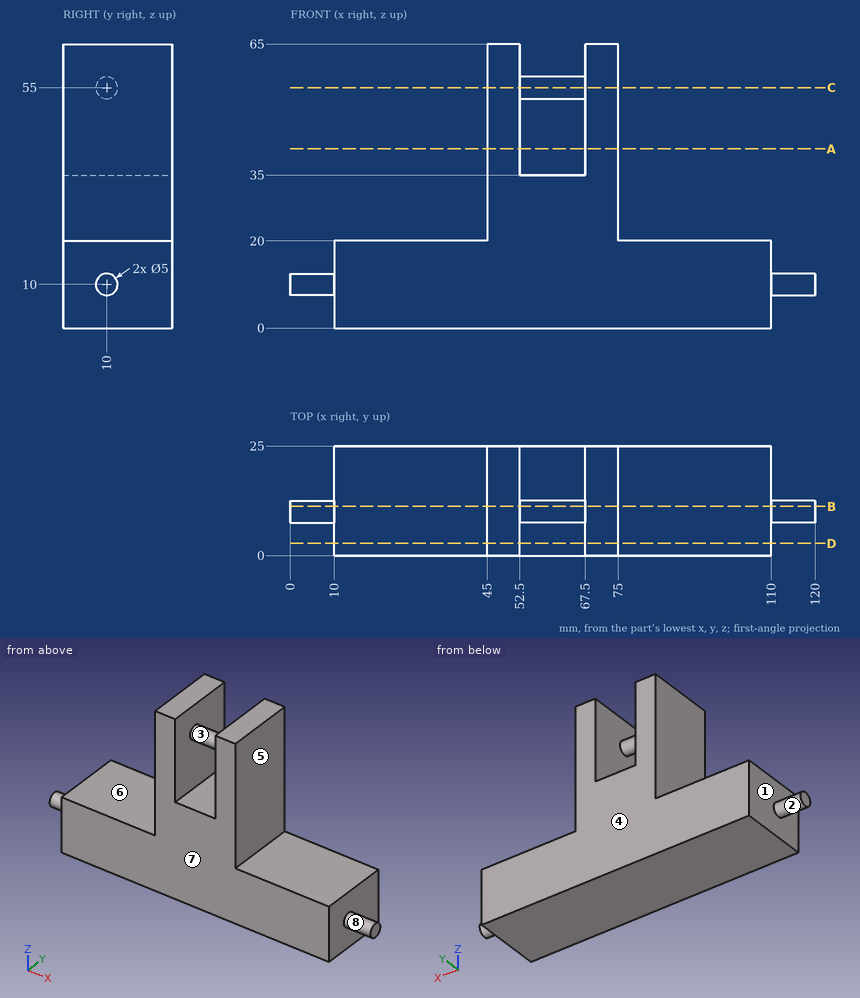
Answer from the drawing. Dimensions are ordinates in mm from the lowest x, y and z of the part. A direction names the side the tool comes from. Give positions to 0.01 mm unless a question says otherwise; leave off trailing zeros. Order: outer loops, then holes, each group sorted by start corner. A loop starts at its lowest first (then second) coordinate and runs counter-clockwise, first axis right, second up.
(1) Find section A-A (z = 41). Give the vertices of the cut face in (x, y), plus the area to 3 significant figures.
(2) Given pin 1 (7.5 mm diameter, centred on x = 19.5, y = 12.5, fed in from +Z); pin 2 (10 mm diameter, centred on y = 4.5, z = 43.5, fed in from +X); pin 3 (12.5 mm diameter, centred on y = 7.5, z = 49, fed in from -X), each flat-ended and moving along its own axis, determine where each tip first touches the part or whether it passes through.
(3) For the marked faces 4, 5, 6, 7 and 8, determine the directions among +Z, -Z, +X, -X, +Y, -Y from which every point of the face is accessible in a straight line to the end or side of a thin tool.
(4) Find section C-C (z = 55). Give the vertices of the cut face in (x, y).
(5) Find section D-D (y = 2.75). Give the vertices of the cut face in (x, z).
(6) Straight lines are drawn through the part: L1, parallel to X at y = 11.25, z = 49.5; L2, parallel to Z at x = 78, y = 7.25; L3, parallel to X at y = 20.75, z = 29.5. For each, find the intervals that lie inside material, in ascending order.
(7) For a pull along X with two mould halves and no side action, classify the marked faces 1, 2 and 3 as released by +X, released by -X, zero draft, split by the parting line, or undercut.
(8) Find section B-B (y = 11.25). Give the vertices of the cut face in (x, z), plus the area to 3 significant figures.
Result sheet:
1. outline: (45, 0) - (52.5, 0) - (52.5, 25) - (45, 25) - close; (67.5, 0) - (75, 0) - (75, 25) - (67.5, 25) - close
1. area: 375 mm2
2. pin 1: stops at z = 20
2. pin 2: stops at x = 75
2. pin 3: stops at x = 45
3. face 4: +Z, -Z, +X, -X, +Y
3. face 5: +Z, +X, +Y, -Y
3. face 6: +Z, -X, +Y, -Y
3. face 7: +Z, -Z, +X, -X, -Y
3. face 8: +X
4. outline: (45, 0) - (52.5, 0) - (52.5, 7.5) - (67.5, 7.5) - (67.5, 0) - (75, 0) - (75, 25) - (67.5, 25) - (67.5, 12.5) - (52.5, 12.5) - (52.5, 25) - (45, 25) - close
5. outline: (10, 0) - (110, 0) - (110, 20) - (75, 20) - (75, 65) - (67.5, 65) - (67.5, 35) - (52.5, 35) - (52.5, 65) - (45, 65) - (45, 20) - (10, 20) - close
6. L1: x = 45 to 52.5, 67.5 to 75
6. L2: z = 0 to 20
6. L3: x = 45 to 75
7. face 1: released by -X
7. face 2: zero draft
7. face 3: undercut
8. outline: (0, 7.83) - (10, 7.83) - (10, 0) - (110, 0) - (110, 7.83) - (120, 7.83) - (120, 12.17) - (110, 12.17) - (110, 20) - (75, 20) - (75, 65) - (67.5, 65) - (67.5, 57.17) - (52.5, 57.17) - (52.5, 65) - (45, 65) - (45, 20) - (10, 20) - (10, 12.17) - (0, 12.17) - close; hole (52.5, 35) - (67.5, 35) - (67.5, 52.83) - (52.5, 52.83) - close
8. area: 3,050 mm2
